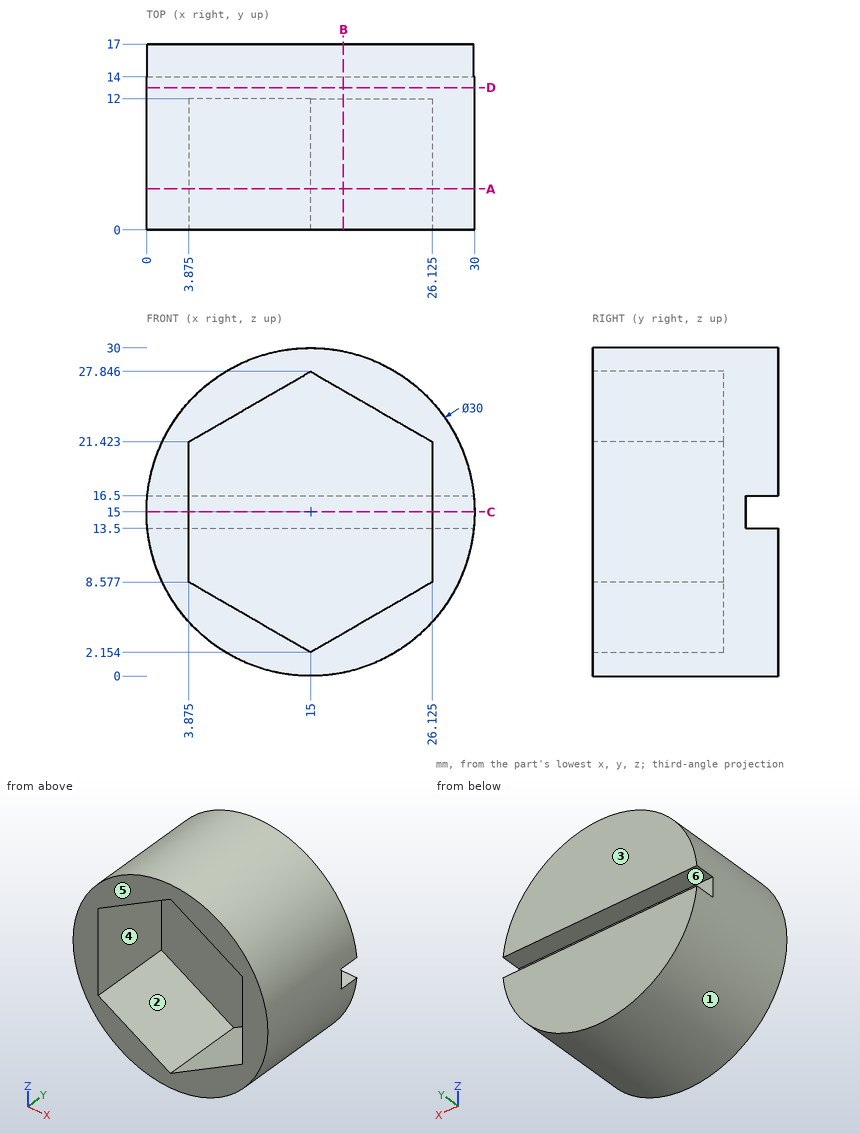
Geometry: see drawing. Coordinates: mm, zero at the bounding-box minimum. A direction names the side the tool comes from. Give positions to 0.01 mm unless a question says otherwise; leave off trailing zeros. Loops run counter-clockwise (first coordinate to the right, second up) from the corner with the lowest first, then second, coordinate; pieces in that order, holes last. Notation, with made-up numbers: (-12, -33) -> (-4, -33) arc R15 ccw to (-4, -22) -> close; hole circle Ø9 at (28, 45.5). An arc over 180 degrees is marked (long way). Answer as a JSON object with one key per item and string values. Group by question number.
Item 1: Cut plane B-B, the plane x = 18. Return the cut outline in (y, z).
Item 2: Cut plane D-D, the plane y = 13. Return the cut outline in (x, z), and give its area (3 significant figures).
Item 3: Cut plane C-C, the plane z = 15. Return the cut outline in (x, y) (3 decimals).
Item 4: Line query: probe 1 along Z at (x, y) = (15.25, 16); probe 2 along Y at (x, z) = (12.75, 12); probe 3 along Y at (x, z) = (24.75, 15.75). Output: solid intervals per line, ascending.
Item 5: Pin query (flat end, axial travel): P1, Ø3.5, axis at y = 6.5, z = 13.5, coming from the -X side; P2, Ø5, axis at x = 23, y = 4, coming from the -Z side; P3, Ø5, axis at x = 25, y = 5, coming from the +Z side; P4, Ø6, axis at x = 26.5, y = 9, coming from the -Z side. Return the tip coordinate at first contact, or that it passes through.
Item 6: Reachability of the marked faces 4, 5 and 6 from +Z, -Z, +X, -X, +Y, -Y: full face, straight path, thin tool, end or side. Return the list, or none.
Item 7: Pull-direction query (Z, two-part tool) for the marked faces 1, 2 and 3; classes: released by +Z, released by -Z, zero draft, split by the parting line, or undercut.
Item 8: Cut plane A-A, the plane y = 3.75. Return the cut outline in (x, z) (3 decimals), and give its area (3 significant figures).
Checks:
{
 "1": {"outline": "(0, 0.3) -> (17, 0.3) -> (17, 13.5) -> (14, 13.5) -> (14, 16.5) -> (17, 16.5) -> (17, 29.7) -> (0, 29.7) -> (0, 26.11) -> (12, 26.11) -> (12, 3.89) -> (0, 3.89) -> close"},
 "2": {"outline": "circle Ø30 at (15, 15)", "area": "707 mm²"},
 "3": {"outline": "(0, 0) -> (3.875, 0) -> (3.875, 12) -> (26.125, 12) -> (26.125, 0) -> (30, 0) -> (30, 14) -> (0, 14) -> close"},
 "4": {"probe 1": "z = 0 to 13.5, 16.5 to 30", "probe 2": "y = 12 to 17", "probe 3": "y = 12 to 14"},
 "5": {"P1": "stops at x = 0", "P2": "stops at z = 1.04", "P3": "stops at z = 27.99", "P4": "stops at z = 2.64"},
 "6": {"face 4": "-Y", "face 5": "+Z, -Z, +X, -X, -Y", "face 6": "+X, -X, +Y"},
 "7": {"face 1": "split by the parting line", "face 2": "undercut", "face 3": "zero draft"},
 "8": {"outline": "circle Ø30 at (15, 15); hole (3.875, 8.577) -> (15, 2.154) -> (26.125, 8.577) -> (26.125, 21.423) -> (15, 27.846) -> (3.875, 21.423) -> close", "area": "278 mm²"}
}
